```python
from build123d import *

# Parameters (mm, degrees)
SKIZZE1_R                                 = 11.5
GRUNDK_RPER_WALZE_DEPTH                   = 74
PRESSPASSUNG_KUGELLAGER_DEPTH             = 4.3
SKIZZE3_R                                 = 2.25
M4_SCHRAUBENF_HRUNG_DEPTH                 = 4.5
SKIZZE4_R                                 = 9.675
MOTORAUSSPARUNG_DEPTH                     = 12.75
ZERST_RUNGSELEMENT_START                  = -6
SKIZZE7_W                                 = 1.5
SKIZZE7_H                                 = 15
ZERST_RUNGSELEMENT_AUSSPARUNG_DEPTH       = 63
SKIZZE8_W                                 = 63
SKIZZE8_H                                 = 4
ZERST_RUNGSELEMENT_RECHTECK_DEPTH         = 1.5
M5_MOTOR_MUTTER_DEPTH                     = 12
SKIZZE12_R                                = 3.1
M5_AUSLAUF_SCHRAUBE_DEPTH                 = 2
ZERST_RUNGSELEMENT_VERVIELF_LTIGUNG_COUNT = 5
FASE1_SIZE                                = 0.4


with BuildPart() as part:
    # Skizze1 → Grundkörper Walze (new body)
    with BuildSketch(Plane(origin=(0, 0, 0), x_dir=(0, 0, -1), z_dir=(1, 0, 0))):
        Circle(SKIZZE1_R)
    extrude(amount=GRUNDK_RPER_WALZE_DEPTH)

    # Skizze2 → Presspassung Kugellager (cut)
    with BuildSketch(Plane(origin=(74, 0, 0), x_dir=(0, 0, -1), z_dir=(1, 0, 0))):
        with BuildLine():
            Line((-7.1137911, 1.5230237), (-7.0137911, 1.5230237))
            Line((-7.0137911, 1.5230237), (-7.0137911, -1.4769763))
            Line((-7.0137911, -1.4769763), (-7.123493947, -1.4769763))
            ThreePointArc((-7.123493947, -1.4769763), (-5.899398016, -4.257079756), (-3.646763959, -6.294977175))
            Line((-3.646763959, -6.294977175), (-3.61586226, -6.199871523))
            Line((-3.61586226, -6.199871523), (-0.762692711, -7.126922506))
            Line((-0.762692711, -7.126922506), (-0.796592755, -7.231256114))
            ThreePointArc((-0.796592755, -7.231256114), (2.225709199, -6.926170916), (4.859967024, -5.413533553))
            Line((4.859967024, -5.413533553), (4.779065325, -5.354755027))
            Line((4.779065325, -5.354755027), (6.542421081, -2.927704044))
            Line((6.542421081, -2.927704044), (6.631172549, -2.99218576))
            ThreePointArc((6.631172549, -2.99218576), (7.27496195, -0.023529282), (6.650388764, 2.94922944))
            Line((6.650388764, 2.94922944), (6.569487065, 2.890450915))
            Line((6.569487065, 2.890450915), (4.806131308, 5.317501898))
            Line((4.806131308, 5.317501898), (4.894882775, 5.381983613))
            ThreePointArc((4.894882775, 5.381983613), (2.270464553, 6.91162902), (-0.749800729, 7.236257587))
            Line((-0.749800729, 7.236257587), (-0.71889903, 7.141151935))
            Line((-0.71889903, 7.141151935), (-3.572068579, 6.214100952))
            Line((-3.572068579, 6.214100952), (-3.605968623, 6.31843456))
            ThreePointArc((-3.605968623, 6.31843456), (-5.871737686, 4.295150934), (-7.1137911, 1.5230237))
        make_face()
    extrude(amount=-PRESSPASSUNG_KUGELLAGER_DEPTH, mode=Mode.SUBTRACT)

    # Skizze3 → M4 Schraubenführung (cut)
    with BuildSketch(Plane(origin=(69.7, 0, 0), x_dir=(0, 0, -1), z_dir=(1, 0, 0))):
        Circle(SKIZZE3_R)
    extrude(amount=-M4_SCHRAUBENF_HRUNG_DEPTH, mode=Mode.SUBTRACT)

    # Skizze4 → Motoraussparung (cut)
    with BuildSketch(Plane.ZY):
        Circle(SKIZZE4_R)
    extrude(amount=-MOTORAUSSPARUNG_DEPTH, mode=Mode.SUBTRACT)

    # Skizze7 → Zerstörungselement Aussparung (cut)
    with BuildSketch(Plane(origin=(74, 0, 0), x_dir=(0, 0, -1), z_dir=(1, 0, 0)).offset(ZERST_RUNGSELEMENT_START)):
        with Locations((-10.75, 0)):
            Rectangle(SKIZZE7_W, SKIZZE7_H)
    zerst_rungselement_aussparung = extrude(amount=-ZERST_RUNGSELEMENT_AUSSPARUNG_DEPTH, mode=Mode.SUBTRACT)

    # Skizze8 → Zerstörungselement Rechteck (add)
    with BuildSketch(Plane.XY.offset(10)):
        with Locations((36.5, 0)):
            Rectangle(SKIZZE8_W, SKIZZE8_H)
    zerst_rungselement_rechteck = extrude(amount=ZERST_RUNGSELEMENT_RECHTECK_DEPTH)

    # Skizze10 → M5 Motor Mutter (cut)
    with BuildSketch(Plane.ZY.offset(-12.75)):
        Polygon((4.139835299, -2.29675794), (4.058968371, 2.436823566), (-0.080866927, 4.733581506), (-4.139835299, 2.29675794), (-4.058968371, -2.436823566), (0.080866927, -4.733581506), align=None)
    extrude(amount=-M5_MOTOR_MUTTER_DEPTH, mode=Mode.SUBTRACT)

    # Skizze12 → M5 Auslauf Schraube (cut)
    with BuildSketch(Plane.ZY.offset(-24.75)):
        Circle(SKIZZE12_R)
    extrude(amount=-M5_AUSLAUF_SCHRAUBE_DEPTH, mode=Mode.SUBTRACT)

    # Zerstörungselement Vervielfältigung: Zerstörungselement Aussparung, Zerstörungselement Rechteck ×5 about axis
    zerst_rungselement_vervielf_ltigung_axis = Axis((0, 0, 0), (1, 0, 0))
    add([zerst_rungselement_aussparung.rotate(zerst_rungselement_vervielf_ltigung_axis, i * 360 / ZERST_RUNGSELEMENT_VERVIELF_LTIGUNG_COUNT) for i in range(1, ZERST_RUNGSELEMENT_VERVIELF_LTIGUNG_COUNT)], mode=Mode.SUBTRACT)
    add([zerst_rungselement_rechteck.rotate(zerst_rungselement_vervielf_ltigung_axis, i * 360 / ZERST_RUNGSELEMENT_VERVIELF_LTIGUNG_COUNT) for i in range(1, ZERST_RUNGSELEMENT_VERVIELF_LTIGUNG_COUNT)])

    # Skizze15 → Innenaussparung (revolve, cut)
    with BuildSketch(Plane.XY, mode=Mode.PRIVATE) as innenaussparung_sk:
        Polygon((27.25, 0), (35.75, 8.5), (65.2, 8.5), (65.2, 0), align=None)
    revolve(innenaussparung_sk.sketch.rotate(Axis((-6.893942049, 0, 0), (1, 0, 0)), 90), axis=Axis((-6.893942049, 0, 0), (1, 0, 0)), mode=Mode.SUBTRACT)

    # Fase1
    fase1_edges = [part.edges().sort_by_distance(p)[0] for p in [
        (0, 0, -9.675),
    ]]
    chamfer(fase1_edges, length=FASE1_SIZE)


solid = part.part
```
Check sheet for the modelled part. Datum: model origin and axes. Units: mm. A direction names the side the tool comes from. Coordinates: 2 decimals unless noted, no trailing zeros. Write item = value, one per line. Start each with the question number.
1. Thickness scan on probe 1 along Z at (x, y) = (61.5, 1.5); probe 2 along Y at (x, z) = (68.75, 0); probe 3 along X at (y, z) = (-4.5, -10.25). Record the ranges inside material, lowest first.
2. Mould release check, pull along Y, two halves, no side actions. Record for faces 1 (the flat face through (68, -11, 0)), 2 (the flat face through (36.941, -10.705, -0.586)), 3 (the flat face through (71.88, -6.657, 2.209)), 4 (the cylindrical face through (71.88, 4.33, 5.846)): pulls with the +Y half, pulls with the -Y half, needs draft (parallel to the pull), parting line crosses it, or undercut.
3. Go/stop test with flat-tipped pins: pin 1 (5 mm diameter, centred on y = 0, z = 0, fed in from +X); pin 2 (0.8 mm diameter, centred on x = 32, z = 10.5, fed in from +Y); pin 3 (0.7 mm diameter, centred on y = 4.5, z = 11, fed in from -X); pin 4 (10 mm diameter, centred on y = -1.5, z = 1.5, fed in from -X). Record where each tip stops, or that it passes through.
4. Tool access check on faces 5 (the flat face through (71.88, 4.09, -5.7)), 6 (the flat face through (12.75, -4, 2)), 7 (the flat face through (5, 11, 0)), 8 (the flat face through (5, -9, -6.5)). Record the directions out of +Z, -Z, +X, -X, +Y, -Y that give a thin tool (end or side, any length) a straight path to the whole face; none if there is none.
The answers:
q1.probe_1 = -11.27 to -8.37, 8.37 to 11.5
q1.probe_2 = -11.5 to -2.25, 2.25 to 11.5
q1.probe_3 = 0 to 5, 68 to 74
q2.face_1 = needs draft
q2.face_2 = pulls with the -Y half
q2.face_3 = undercut
q2.face_4 = undercut
q3.pin_1 = 69.7
q3.pin_2 = 2
q3.pin_3 = through
q3.pin_4 = 12.75
q4.face_5 = +X
q4.face_6 = -X
q4.face_7 = +Y
q4.face_8 = -Y
